Work out the finished part from the listing and answer in its coordinate system (mm). A direction names the side the tool comes from. Round coordinates to 2 decimals unless told otherwise and drop trailing zeros. Loops run counter-clockwise (first coordinate to the right, second up) from the corner with the lowest first, then second, coordinate; pieces in that order, holes last. Notation, with made-up numbers: (52, 0.25) -> (80, 0.25) arc R34 ccw to (80, 30.25) -> close; hole circle Ø6 at (88.5, 15). An arc over 180 degrees is marked (long way). Use one line per item in the form item = value.
```python
from build123d import *

# Parameters (mm, degrees)
SKETCH_1_W               = 40
SKETCH_1_H               = 40
EXTRUDE_1_DEPTH          = 40
SKETCH_2_W               = 25
SKETCH_2_H               = 40
CUT_EXTRUDE_1_DEPTH      = 34
SKETCH_3_R               = 2.5
CUT_EXTRUDE_2_DEPTH      = 7
CHAMFER_1_SIZE           = 5
SKETCH_5_R               = 12
CUT_EXTRUDE_4_DEPTH      = 8
CUT_EXTRUDE_5_REACH      = 34
SKETCH_7_R               = 10
CUT_EXTRUDE_6_REACH      = 42
SKETCH_4_R               = 11
SKETCH_9_R               = 1.5
CUT_EXTRUDE_7_DEPTH      = 41
PATTERN_CIRCULAR_1_COUNT = 4


with BuildPart() as part:
    # 草圖1 → 填料-伸長1 (new body)
    with BuildSketch(Plane.XY):
        Rectangle(SKETCH_1_W, SKETCH_1_H)
    extrude(amount=EXTRUDE_1_DEPTH)

    # 草圖2 → 除料-伸長1 (cut)
    with BuildSketch(Plane.XY.offset(40)):
        with Locations((2.5, 0)):
            Rectangle(SKETCH_2_W, SKETCH_2_H)
    extrude(amount=-CUT_EXTRUDE_1_DEPTH, mode=Mode.SUBTRACT)

    # 草圖3 → 除料-伸長2 (cut, through all)
    with BuildSketch(Plane.XY.offset(6)):
        with Locations((0, 10)):
            Circle(SKETCH_3_R)
        with Locations((0, -10)):
            Circle(SKETCH_3_R)
    extrude(amount=-CUT_EXTRUDE_2_DEPTH, mode=Mode.SUBTRACT)

    # 導角1
    chamfer_1_edges = [part.edges().sort_by_distance(p)[0] for p in [
        (-15, -20, 40),
        (-15, 20, 40),
        (17.5, -20, 40),
        (17.5, 20, 40),
    ]]
    chamfer(chamfer_1_edges, length=CHAMFER_1_SIZE)

    # 草圖5 → 除料-伸長4 (cut)
    with BuildSketch(Plane.ZY.offset(20)):
        with Locations((20, 0)):
            Circle(SKETCH_5_R)
    extrude(amount=-CUT_EXTRUDE_4_DEPTH, mode=Mode.SUBTRACT)

    # 草圖7 → 除料-伸長5 (cut, up to next)
    with BuildSketch(Plane.ZY.offset(12), mode=Mode.PRIVATE) as cut_extrude_5_sk1:
        with Locations((20, 0)):
            Circle(SKETCH_7_R)
    cut_extrude_5_tool1 = extrude(cut_extrude_5_sk1.sketch, amount=-CUT_EXTRUDE_5_REACH, mode=Mode.PRIVATE) & part.part
    add(cut_extrude_5_tool1.solids().sort_by_distance((-12, 0, 20))[0], mode=Mode.SUBTRACT)

    # 草圖4 → 除料-伸長6 (cut, up to next)
    with BuildSketch(Plane(origin=(20, 0, 0), x_dir=(0, 0, -1), z_dir=(1, 0, 0)), mode=Mode.PRIVATE) as cut_extrude_6_sk1:
        with Locations((-20, 0)):
            Circle(SKETCH_4_R)
    cut_extrude_6_tool1 = extrude(cut_extrude_6_sk1.sketch, amount=-CUT_EXTRUDE_6_REACH, mode=Mode.PRIVATE) & part.part
    add(cut_extrude_6_tool1.solids().sort_by_distance((20, 0, 20))[0], mode=Mode.SUBTRACT)

    # 草圖9 → 除料-伸長7 (cut, through all)
    with BuildSketch(Plane(origin=(20, 0, 0), x_dir=(0, 0, -1), z_dir=(1, 0, 0))):
        with Locations((-9.393398282, 10.606601718)):
            Circle(SKETCH_9_R)
    cut_extrude_7 = extrude(amount=-CUT_EXTRUDE_7_DEPTH, mode=Mode.SUBTRACT)

    # 環狀複製排列1: 除料-伸長7 ×4 about axis
    pattern_circular_1_axis = Axis((0, 0, 20), (1, 0, 0))
    for i in range(1, PATTERN_CIRCULAR_1_COUNT):
        add(cut_extrude_7.rotate(pattern_circular_1_axis, i * 360 / PATTERN_CIRCULAR_1_COUNT), mode=Mode.SUBTRACT)


solid = part.part
```
(1) For a pull along Z with two mould halves and no side action, classify faces 5 (the flat face through (0, 0, 0)), 6 (the cylindrical face through (17.535, 10.281, 29.142)), 7 (the flat face through (-15, 17, 38)) as +Z half, -Z half, draft (parallel to the pull), parting line (faces both ways), or undercut.
Completed:
face_5 = -Z half
face_6 = undercut
face_7 = +Z half
(2) Find section B-B, the plane y = 0. Write down the section's boundary in (x, z).
Completed:
outline = (-20, 0) -> (20, 0) -> (20, 9) -> (15, 9) -> (15, 6) -> (-10, 6) -> (-10, 10) -> (-12, 10) -> (-12, 8) -> (-20, 8) -> close; (-20, 32) -> (-12, 32) -> (-12, 30) -> (-10, 30) -> (-10, 40) -> (-20, 40) -> close; (15, 31) -> (20, 31) -> (20, 40) -> (15, 40) -> close
(3) Find section D-D, the plane y = 16.5. Write down the section's boundary in (x, z).
Completed:
outline = (-20, 0) -> (20, 0) -> (20, 38.5) -> (15, 38.5) -> (15, 6) -> (-10, 6) -> (-10, 38.5) -> (-20, 38.5) -> close
(4) Given P1, Ø8, axis at x = 0, y = -10, coming from the +Z side; P2, Ø1.8, axis at y = 10.61, z = 30.61, coming from the +X side, each flat-ended and moving along its own axis, determine where each tip first touches the part or whether it passes through.
Completed:
P1 = 6
P2 = through
(5) For faces 1 (the cylindrical face through (-14.93, 10.281, 29.142)), 2 (the flat face through (-12, 9, 15)), 3 (the cylindrical face through (17.535, -4.213, 9.839)), 4 (the flat face through (15, 4, 31)), determine the directions among +Z, -Z, +X, -X, +Y, -Y from which every point of the face is accessible in a straight line to the end or side of a thin tool.
Completed:
face_1 = +X, -X
face_2 = -X
face_3 = +X
face_4 = +Z, +Y, -Y
(6) Consider L1, parallel to Y at x = 0, z = 4.5; L2, parallel to X at y = 14.5, z = 20; L3, parallel to X at y = 2, z = 8.5. Determine where each line is inside the solid, lowest interval first.
Completed:
L1 = -20 to -12.5, -7.5 to 7.5, 12.5 to 20
L2 = -20 to -10, 15 to 20
L3 = -12 to -10, 15 to 20
(7) Find section A-A, the plane z = 20. Write down the section's boundary in (x, y), then the cut area to 3 significant figures.
Completed:
outline = (-20, -20) -> (-10, -20) -> (-10, -10) -> (-12, -10) -> (-12, -12) -> (-20, -12) -> close; (-20, 12) -> (-12, 12) -> (-12, 10) -> (-10, 10) -> (-10, 20) -> (-20, 20) -> close; (15, -20) -> (20, -20) -> (20, -11) -> (15, -11) -> close; (15, 11) -> (20, 11) -> (20, 20) -> (15, 20) -> close
area = 258 mm2
(8) Find section C-C, the plane x = 0. Write down the section's boundary in (y, z).
Completed:
outline = (-20, 0) -> (-12.5, 0) -> (-12.5, 6) -> (-20, 6) -> close; (-7.5, 0) -> (7.5, 0) -> (7.5, 6) -> (-7.5, 6) -> close; (12.5, 0) -> (20, 0) -> (20, 6) -> (12.5, 6) -> close
